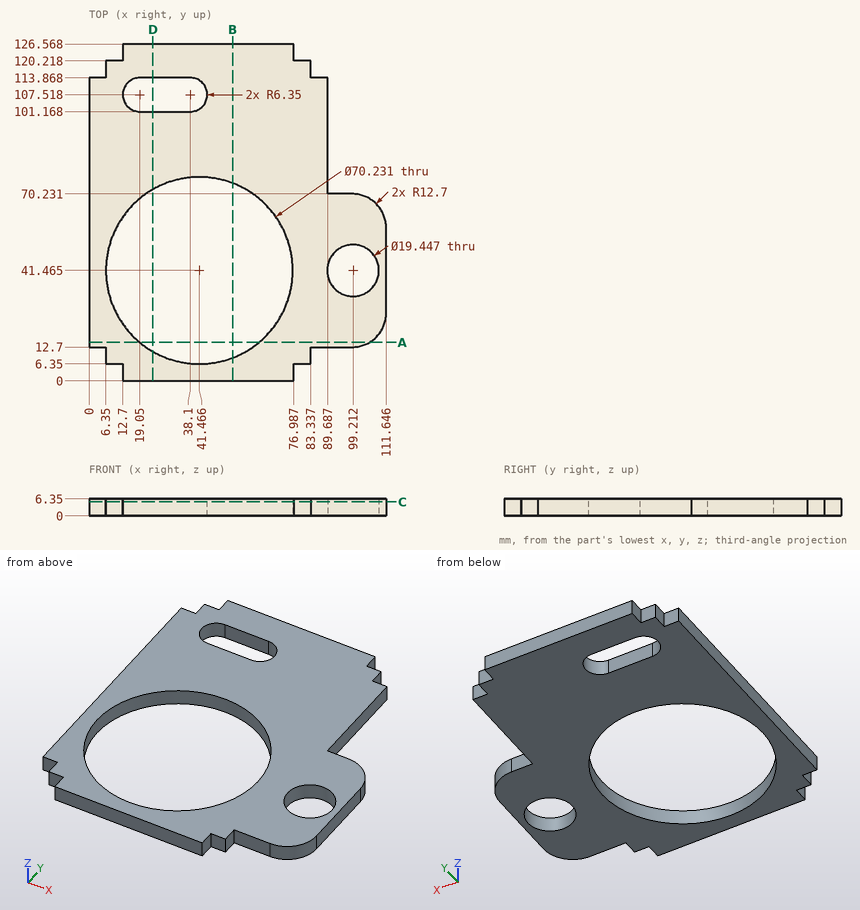
Drawing for the job (mm, zero at the part's lowest x, y, z). Round coordinates to 2 decimals unless told otherwise and drop trailing zeros. Write each loop counter-clockwise with the first axis right and the second up, starting at its lowest first coordinate (ties: lowest second). Pieces come first, ordered by that corner, then holes. Notation, with made-up numbers: (-14.75, -25) - (3.25, -25) arc R10 cw to (3.25, -8) - close; hole circle Ø3 at (-6, 27). An arc over 180 degrees is marked (long way). Return JSON: item names as keys, results as strings. Group by question number.
Item 1: Band-saw the part on D-D on x = 24. List the corners of the cut face in (y, z), plus the area to 3 significant figures.
Item 2: Flat gauge pins, fed straight in: pin 1 Ø3 at (y, z) = (3, 3) entering from +X; pin 2 Ø3 at (y, z) = (116.5, 2) entering from -X; pin 3 Ø3 at (x, z) = (86, 4) entering from -Y. Where does each tip first touch, or does it go through?
Item 3: Band-saw the part on C-C on z = 5.25. State how many separate pieces and enclosed holes the cut face has, plus the area to 3 significant figures.
Item 4: Probe probe 1 along X at (y, z) = (42, 0.5) (1 decimal); probe 2 along Y at (x, z) = (39.5, 4) (1 decimal); probe 3 along Y at (x, z) = (20, 2.5) (1 decimal). List the from-to ranges inside material, lowest first.
Item 5: Band-saw the part on B-B on x = 54. List the corners of the cut face in (y, z).
Item 6: Band-saw the part on A-A on y = 14.5. List the corners of the cut face in (x, z).
Resolved:
{
 "1": {"outline": "(0, 0) - (11, 0) - (11, 6.35) - (0, 6.35) - close; (71.93, 0) - (101.17, 0) - (101.17, 6.35) - (71.93, 6.35) - close; (113.87, 0) - (126.57, 0) - (126.57, 6.35) - (113.87, 6.35) - close", "area": "336 mm²"},
 "2": {"pin 1": "stops at x = 76.99", "pin 2": "stops at x = 6.35", "pin 3": "stops at y = 12.7"},
 "3": {"separate pieces": "1", "enclosed holes": "3", "area": "7,520 mm²"},
 "4": {"probe 1": "x = 0 to 6.4, 76.6 to 89.5, 108.9 to 111.6", "probe 2": "y = 0 to 6.4, 76.5 to 101.3, 113.7 to 126.6", "probe 3": "y = 0 to 13.7, 69.3 to 101.2, 113.9 to 126.6"},
 "5": {"outline": "(0, 0) - (8.66, 0) - (8.66, 6.35) - (0, 6.35) - close; (74.27, 0) - (126.57, 0) - (126.57, 6.35) - (74.27, 6.35) - close"},
 "6": {"outline": "(0, 0) - (18.97, 0) - (18.97, 6.35) - (0, 6.35) - close; (63.96, 0) - (105.46, 0) - (105.46, 6.35) - (63.96, 6.35) - close"}
}
